The listing builds one solid part. Answer for the finished solid, in the listing's coordinates (mm). A direction names the side the tool comes from. Round coordinates to 2 decimals unless told otherwise and drop trailing zeros. Write each loop counter-clockwise with the first axis right and the second up, starting at its lowest first coordinate (ties: lowest second). Pieces come first, ordered by that corner, then holes.
from build123d import *

# Parameters (mm, degrees)
SKETCH_1_R          = 4
EXTRUDE_1_DEPTH     = 7
SKETCH_2_W          = 36
SKETCH_2_H          = 20
EXTRUDE_2_DEPTH     = 36
SKETCH_3_R          = 7.5
CUT_EXTRUDE_2_DEPTH = 36
SKETCH_4_R          = 18
SKETCH_4_R_2        = 7.5
EXTRUDE_3_DEPTH     = 120


with BuildPart() as part:
    # 草图1 → 凸台-拉伸1 (new body)
    with BuildSketch(Plane.XY):
        Polygon((-30, 0), (30, 0), (70, 20), (90, 20), (90, 40), (65.27864045, 40), (25.27864045, 20), (-25.27864045, 20), (-65.27864045, 40), (-90, 40), (-90, 20), (-70, 20), align=None)
        with Locations((80, 30)):
            Circle(SKETCH_1_R, mode=Mode.SUBTRACT)
        with Locations((-80, 30)):
            Circle(SKETCH_1_R, mode=Mode.SUBTRACT)
    extrude(amount=EXTRUDE_1_DEPTH)

    # 草图2 → 凸台-拉伸2 (add)
    with BuildSketch(Plane(origin=(0, 0, 0), x_dir=(-1, 0, 0), z_dir=(0, 0, -1))):
        with Locations((0, 10)):
            Rectangle(SKETCH_2_W, SKETCH_2_H)
    extrude(amount=EXTRUDE_2_DEPTH)

    # 草图3 → 切除-拉伸2 (cut)
    with BuildSketch(Plane(origin=(0, 20, 0), x_dir=(1, 0, 0), z_dir=(0, 1, 0))):
        with BuildLine():
            ThreePointArc((-6.6e-08, 36), (12.727922038, 30.727922085), (18, 18))
            Line((18, 18), (18, 36))
            Line((18, 36), (-6.6e-08, 36))
        make_face()
        with BuildLine():
            Line((-18, 36), (-18, 18))
            ThreePointArc((-18, 18), (-12.727922085, 30.727922038), (-6.6e-08, 36))
            Line((-6.6e-08, 36), (-18, 36))
        make_face()
        with Locations((0.255418615, 18)):
            Circle(SKETCH_3_R)
    extrude(amount=-CUT_EXTRUDE_2_DEPTH, mode=Mode.SUBTRACT)

    # 草图4 → 凸台-拉伸3 (add)
    with BuildSketch(Plane(origin=(0, 20, 0), x_dir=(1, 0, 0), z_dir=(0, 1, 0))):
        with Locations((0.255418615, 18)):
            Circle(SKETCH_4_R)
        with Locations((0.255418615, 18)):
            Circle(SKETCH_4_R_2, mode=Mode.SUBTRACT)
    extrude(amount=EXTRUDE_3_DEPTH)


solid = part.part
1. For a pull along X with two mould halves and no side action, classify faces 6 (the face through (0, 140, -10)), 7 (the face through (79.479, 33.966, 3.451)), 8 (the face through (45.56, 30.14, 3.45)), 9 (the face through (-50, 10, 3)) as released by +X, released by -X, zero draft, split by the parting line, or undercut.
Geometry says:
face 6: zero draft
face 7: undercut
face 8: undercut
face 9: released by -X
2. Section A-A on y = 14.5 is taken. Determine the outline of the cut face in (x, z), plus the area to 3 significant figures.
Geometry says:
outline: (-59, 0) - (-18, 0) - (-18, -18) arc R18 ccw to (18, -18) - (18, 0) - (59, 0) - (59, 7) - (-59, 7) - close; hole circle Ø15 at (0.26, -18)
area: 1,810 mm2
3. Section D-D on z = -13 is taken. Determine the outline of the cut face in (x, y), plus the area to 3 significant figures.
Geometry says:
outline: (-18, 0) - (-5.33, 0) - (-5.33, 140) - (-17.04, 140) - (-17.04, 20) - (-18, 20) - close; (5.85, 0) - (18, 0) - (18, 20) - (17.55, 20) - (17.55, 140) - (5.85, 140) - close
area: 3,300 mm2
4. Given pin 1 (7.5 mm diameter, centred on x = 84.5, z = 3, fed in from -Y); pin 2 (2 mm diameter, centred on x = 77.5, z = 2, fed in from +Y); pin 3 (2 mm diameter, centred on y = 124.5, z = -10.5, fed in from -X), each flat-ended and moving along its own axis, determine where each tip first touches the part or whether it passes through.
Geometry says:
pin 1: stops at y = 20
pin 2: stops at y = 40
pin 3: stops at x = -16.53
5. Straight lines are drawn through the part: line 1 along X through (y, z) = (68, -18); line 2 along Y through (x, z) = (-80, 2); line 3 along Z through (x, y) = (73, 37.5). For each, find the intervals that lie inside material, in ascending order.
Geometry says:
line 1: x = -17.74 to -7.24, 7.76 to 18.26
line 2: y = 20 to 26, 34 to 40
line 3: z = 0 to 7
6. Section C-C on y = 30 is taken. Determine the outline of the cut face in (x, z), plus the area to 3 significant figures.
Geometry says:
outline: (-90, 0) - (-84, 0) - (-84, 7) - (-90, 7) - close; (-76, 0) - (-45.28, 0) - (-45.28, 7) - (-76, 7) - close; circle Ø36 at (0.26, -18); (45.28, 0) - (76, 0) - (76, 7) - (45.28, 7) - close; (84, 0) - (90, 0) - (90, 7) - (84, 7) - close; hole circle Ø15 at (0.26, -18)
area: 1,360 mm2
7. A tool of negligible diameter and unlimited length cuts with its end or side. For faces 1 (the face through (-3.65, 79.16, -0.43)), 2 (the face through (-45, 29.86, 3.45)), 3 (the face through (78, 40, 3)), 4 (the face through (-80, 20, 3)), 5 (the face through (-55, 20, 0)), from which of +Z, -Z, +X, -X, +Y, -Y can it reach the whole face along a straight path? Write none if from no direction.
Geometry says:
face 1: +Y
face 2: +Z, -Z, +Y
face 3: +Z, -Z, +X, -X, +Y
face 4: +Z, -Z, -X, -Y
face 5: -Z, -X, +Y, -Y
8. Section B-B on x = 80 is taken. Determine the outline of the cut face in (y, z).
Geometry says:
outline: (20, 0) - (26, 0) - (26, 7) - (20, 7) - close; (34, 0) - (40, 0) - (40, 7) - (34, 7) - close
